Work out the finished part from the listing and answer in its coordinate system (mm). A direction names the side the tool comes from. Coordinates: 2 decimals unless noted, no trailing zeros. Loops run counter-clockwise (first coordinate to the right, second up) from the corner with the lowest first, then second, coordinate; pieces in that order, holes last. Notation, with made-up numbers: (50.25, 38.5) - (106.25, 38.5) arc R16 cw to (106.25, 61.5) - close; hole circle Ø6 at (10.25, 23). An arc over 180 degrees is marked (long way). Write each question's results on one line, items separated by ' | '. Start each with the question number.
Item 1: Section B-B, the plane y = 316.5 is taken. Write down the section's boundary in (x, z) (3 decimals), plus the area to 3 significant figures.
Item 2: Each of these flat-tipped pins is pushed along its axis until it touches: pin 1 Ø10 at (x, z) = (-28.5, -14.5) entering from -Y; pin 2 Ø7.5 at (x, y) = (-38.1, 511.175) entering from +Z (3 decimals); pin 3 Ø12 at (x, y) = (-20, 442) entering from -Z (3 decimals). Where does it stop, or does it pass through?
Item 3: For a pull along X with two mould halves and no side action, classify faces 6 (the face through (-25, 0, -2)), 7 (the face through (0, 261, -2)), 8 (the face through (-3.175, 13, -13)) as +X half, -X half, draft (parallel to the pull), parting line (faces both ways), or undercut.
Item 4: A tool of negligible diameter and unlimited length cuts with its end or side. For faces 1 (the face through (-38.38, 517.52, -1.61)), 2 (the face through (-25, 511, -22.225)), 3 (the face through (-25, 523.875, -2)), 4 (the face through (-25.3, 498.475, -22.5)), 5 (the face through (-25, 258, 0)), from which of +Z, -Z, +X, -X, +Y, -Y can it reach the whole face along a straight path? Write none if from no direction.
Item 5: Consider probe 1 along Y at (x, z) = (-38.1, -1.65) (3 decimals); probe 2 along X at (y, z) = (12.7, -1.75); probe 3 along Y at (x, z) = (-38.1, -23.3) (3 decimals). Determine where each line is inside the solid, lowest interval first. Write a range as [from, to].
Item 6: Section A-A, the plane z = -8.25 is taken. Write down the section's boundary in (x, y) (3 decimals).
Autodesk Inventor part; units mm, degrees
ref_plane "YZ Plane" through (0, 0, 0) normal (1, 0, 0) x (0, 1, 0)
ref_plane "XZ Plane" through (0, 0, 0) normal (0, 1, 0) x (-1, 0, 0)
ref_plane "XY Plane" through (0, 0, 0) normal (0, 0, 1) x (1, 0, 0)
sketch "Sketch1" plane through (0, 0, 0) normal (0, 1, 0) x (-1, 0, 0)
  line L0 (0, 0) -> (50.8, 0)
  line L1 (50.8, 0) -> (50.8, -25.4)
  line L2 (50.8, -25.4) -> (0, -25.4)
  line L3 (0, -25.4) -> (0, 0)
  line L4 (47.625, -3.175) -> (3.175, -3.175)
  line L5 (3.175, -3.175) -> (3.175, -22.225)
  line L6 (3.175, -22.225) -> (47.625, -22.225)
  line L7 (47.625, -22.225) -> (47.625, -3.175)
  dimension "d0" = 50.8
  dimension "d1" = 25.4
  dimension "d2" = 3.175
extrude "Extrusion1" add sketch "Sketch1" along normal blind 523.875
sketch "Sketch2" plane through (0, 0, 0) normal (1, 0, 0) x (0, 0, -1)
  line L0 (25.4, 0) -> (0, 0)
  line L1 (25.4, 0) -> (25.4, 523.875)
  line L2 (0, 523.875) -> (25.4, 523.875)
  line L3 (0, 0) -> (0, 523.875)
  line L4 (3.175, 0) -> (3.175, 523.875)
  line L5 (25.4, 0) -> (25.4, 523.875)
  line L6 (3.175, 498.475) -> (25.4, 498.475)
  line L7 (25.4, 498.475) -> (25.4, 25.4)
  line L8 (25.4, 25.4) -> (3.175, 25.4)
  line L9 (3.175, 25.4) -> (3.175, 498.475)
  dimension "d5" = 25.4
  dimension "d6" = 25.4
extrude "Extrusion2" cut sketch "Sketch2" against normal blind 663.575 contours L8 L4 L6 L1
sketch "Sketch3" plane through (-50.8, 0, 0) normal (0, 0, 1) x (1, 0, 0)
  line L0 (50.8, 0) -> (0, 0)
  line L1 (50.8, 0) -> (50.8, 523.875)
  line L2 (0, 523.875) -> (50.8, 523.875)
  line L3 (0, 0) -> (0, 523.875)
  line L4 (47.625, 25.4) -> (3.175, 25.4)
  line L5 (3.175, 0) -> (3.175, 25.4)
  line L6 (47.625, 0) -> (3.175, 0)
  line L7 (47.625, 0) -> (47.625, 25.4)
  line L8 (3.175, 498.475) -> (47.625, 498.475)
  line L9 (47.625, 498.475) -> (47.625, 523.875)
  line L10 (3.175, 523.875) -> (47.625, 523.875)
  line L11 (3.175, 498.475) -> (3.175, 523.875)
  point P0 (12.7, 12.7)
  point P1 (38.1, 12.7)
  point P2 (12.7, 511.175)
  point P3 (38.1, 511.175)
  dimension "d9" = 12.7
  dimension "d10" = 12.7
  dimension "d11" = 12.7
  dimension "d12" = 12.7
  dimension "d13" = 12.7
  dimension "d14" = 12.7
  dimension "d15" = 12.7
  dimension "d16" = 12.7
hole "Hole1" at (-38.1, 12.7, 0) at (-12.7, 12.7, 0) at (-38.1, 511.175, 0) at (-12.7, 511.175, 0) direction (0, 0, -1) diameter 6.35 end through all counterbore diameter 12.7 counterbore depth 6.35
properties part number "OverheadSupportBar.ver1-1111-2020"
Answer key:
1) outline: (-50.8, -3.175) - (0, -3.175) - (0, 0) - (-50.8, 0) - close | area: 161 mm^2
2) pin 1: passes through | pin 2: stops at z = -22.225 | pin 3: stops at z = -3.175
3) face 6: draft | face 7: +X half | face 8: undercut
4) face 1: +Z | face 2: +Y, -Y | face 3: +Z, -Z, +X, -X, +Y | face 4: -Z, +X, -X | face 5: +Z, +X, -X, +Y, -Y
5) probe 1: y = [0, 6.35], [19.05, 504.825], [517.525, 523.875] | probe 2: x = [-50.8, -44.45], [-31.75, -19.05], [-6.35, 0] | probe 3: y = [0, 9.525], [15.875, 25.4], [498.475, 508], [514.35, 523.875]
6) outline: (-50.8, 0) - (-47.625, 0) - (-47.625, 25.4) - (-50.8, 25.4) - close; (-50.8, 498.475) - (-47.625, 498.475) - (-47.625, 523.875) - (-50.8, 523.875) - close; (-3.175, 0) - (0, 0) - (0, 25.4) - (-3.175, 25.4) - close; (-3.175, 498.475) - (0, 498.475) - (0, 523.875) - (-3.175, 523.875) - close
